from build123d import *

# Parameters (mm, degrees)
F1_DEPTH = 20


with BuildPart() as f1:
    # F0 (on Front) → F1 (new body)
    with BuildSketch(Plane.XZ):
        Polygon((0, 86.717134), (0, 0), (40, 0), (26.673388, 21.179436), (31.528226, 21.179436), (18.201613, 42.358872), (23.056451, 42.358872), (9.729839, 63.538307), (14.584677, 63.538307), align=None)
    extrude(amount=F1_DEPTH)

    # F2: F1 across plane


with BuildPart() as f1_1:
    add(f1.part)
    add(f1.part.mirror(Plane.YZ))


solid = f1_1.part
Design review of the part built by this model. Coordinates are the model's own, in mm. A direction names the side the tool comes from. Coordinates: 2 decimals unless noted, no trailing zeros. Loops run counter-clockwise (first coordinate to the right, second up) from the corner with the lowest first, then second, coordinate; pieces in that order, holes last. Notation, with made-up numbers: (29.5, 75) -> (86.5, 75) arc R26 ccw to (86.5, 95) -> close; hole circle Ø9 at (77, 76.5). An arc over 180 degrees is marked (long way). Use a Markdown table: item, result. Add a question column.
Item 1: We need section C-C, the plane z = 9. Write out the cut boundary in (x, y).
Item 2: We need section A-A, the plane y = -4. Write out the cut boundary in (x, z), and give its area (3 significant figures).
Item 3: We need section D-D, the plane x = 25.5. Write out the cut boundary in (y, z).
Item 4: Wall thickness on L1, parallel to Z at x = -13.5, y = -8.5; L2, parallel to Z at x = 18.5, y = -11.75; L3, parallel to X at y = -8.5, z = 9: over which ranges is each line inside the solid? List them lowest first. Write a range as from..to.
Item 5: The part is to be moulded in two halves that separate along Z. For faces 1 (the flat face through (1, 0, 34)), 2 (the flat face through (24.96, -9.86, 31.62)), 3 (the flat face through (7.39, -9.86, 74.97)), 4 (the flat face through (-24.96, -9.86, 31.62)), say which applies: +Z half, -Z half, draft (parallel to the pull), parting line (faces both ways), or undercut.
Item 6: Clearance check with flat-ended pins moving along their axes: P1, Ø4, axis at x = -21.5, y = -12, coming from the -Z side; P2, Ø10, axis at x = -8.5, y = -11.5, coming from the +Z side; P3, Ø8, axis at x = 19, y = -9.5, coming from the +Z side; P4, Ø3, axis at y = -10.5, z = 57, coming from the -X side. State where each tip first meets the part, or that it passes through.
Item 7: We need section B-B, the plane x = -28. Write out the cut boundary in (y, z).
Item 8: Machinability: for faces 5 (the flat face through (-16.486, -9.86, 52.8)), 6 (the flat face through (1, -20, 34)), 7 (the flat face through (29, -10, 21.179)), which of the approach directions +Z, -Z, +X, -X, +Y, -Y give a long, thin tool a straight path to every point of the face, cutting with its end or side? Answer none if there is none.
Numbers:
| question | item | result |
|---|---|---|
| 1 | outline | (-34.34, -20) -> (34.34, -20) -> (34.34, 0) -> (-34.34, 0) -> close |
| 2 | outline | (-40, 0) -> (40, 0) -> (26.67, 21.18) -> (31.53, 21.18) -> (18.2, 42.36) -> (23.06, 42.36) -> (9.73, 63.54) -> (14.58, 63.54) -> (0, 86.72) -> (-14.58, 63.54) -> (-9.73, 63.54) -> (-23.06, 42.36) -> (-18.2, 42.36) -> (-31.53, 21.18) -> (-26.67, 21.18) -> close |
| 2 | area | 3,500 mm^2 |
| 3 | outline | (-20, 0) -> (0, 0) -> (0, 30.76) -> (-20, 30.76) -> close |
| 4 | L1 | z = 0..57.55, 63.54..65.26 |
| 4 | L2 | z = 0..41.88, 42.36..49.6 |
| 4 | L3 | x = -34.34..34.34 |
| 5 | face 1 | draft |
| 5 | face 2 | undercut |
| 5 | face 3 | +Z half |
| 5 | face 4 | undercut |
| 6 | P1 | stops at z = 0 |
| 6 | P2 | stops at z = 81.15 |
| 6 | P3 | stops at z = 55.16 |
| 6 | P4 | stops at x = -14.79 |
| 7 | outline | (-20, 0) -> (0, 0) -> (0, 19.07) -> (-20, 19.07) -> close; (-20, 21.18) -> (0, 21.18) -> (0, 26.79) -> (-20, 26.79) -> close |
| 8 | face 5 | -X, +Y, -Y |
| 8 | face 6 | +Z, -Z, +X, -X, -Y |
| 8 | face 7 | +X, +Y, -Y |
